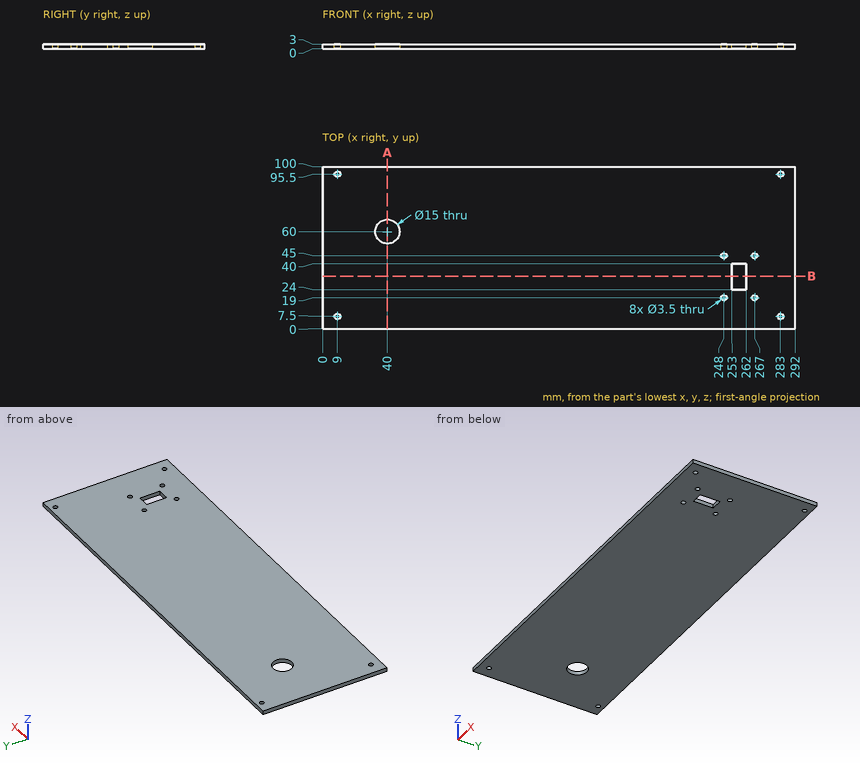
Here's the drawing with two shaded views (mm, measured from the low corner). I have some questions. Coordinates: 2 decimals unless noted, no trailing zeros. Write each loop counter-clockwise with the first axis right and the second up, starting at its lowest first coordinate (ties: lowest second). Pieces come first, ordered by that corner, then holes.
Item 1: Will this pin go through, and if not, where does the flat tip stop? pin 1 (3 mm diameter, centred on x = 283, y = 95.5, fed in from -Z).
Item 2: I want a section at B-B on y = 32.5. Write out the boundary of the cut face in (x, z).
Item 3: If I drill on line 1 (X direction, y = 95.5, z = 2.15); line 2 (Y direction, x = 283, z = 1.5); line 3 (Y direction, x = 40, z = 1.8), over which ranges is the centre line in solid material (lowest first)?
Item 4: I want a section at A-A on x = 40. Write out the boundary of the cut face in (y, z), and give its area (3 significant figures).
Findings below:
1. pin 1: passes through
2. outline: (0, 0) - (253, 0) - (253, 3) - (0, 3) - close; (262, 0) - (292, 0) - (292, 3) - (262, 3) - close
3. line 1: x = 0 to 7.25, 10.75 to 281.25, 284.75 to 292
3. line 2: y = 0 to 5.75, 9.25 to 93.75, 97.25 to 100
3. line 3: y = 0 to 52.5, 67.5 to 100
4. outline: (0, 0) - (52.5, 0) - (52.5, 3) - (0, 3) - close; (67.5, 0) - (100, 0) - (100, 3) - (67.5, 3) - close
4. area: 255 mm2
